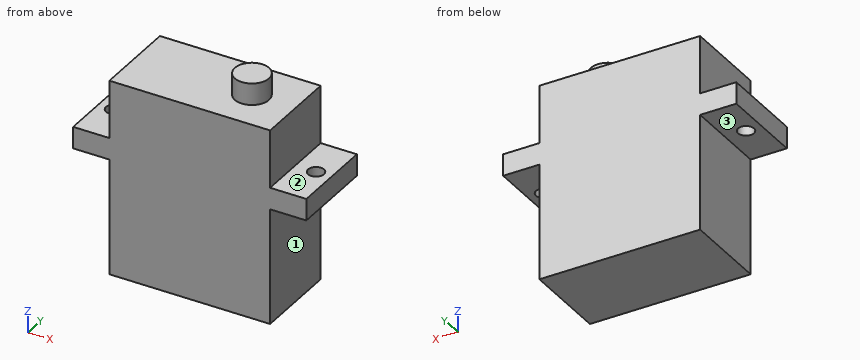
from build123d import *

# Parameters (mm, degrees)
SKETCH1_W           = 32.2
SKETCH1_H           = 11.8
BOSS_EXTRUDE1_DEPTH = 27
SKETCH2_R           = 2.365
BOSS_EXTRUDE2_DEPTH = 3
SKETCH4_W           = 16
SKETCH4_H           = 11.8
CUT_EXTRUDE1_DEPTH  = 5
SKETCH5_W           = 16
SKETCH5_H           = 11.8
CUT_EXTRUDE2_DEPTH  = 5
SKETCH6_W           = 8
SKETCH6_H           = 11.8
CUT_EXTRUDE3_DEPTH  = 5
SKETCH7_W           = 8
SKETCH7_H           = 11.8
CUT_EXTRUDE4_DEPTH  = 5
CUT_EXTRUDE5_REACH  = 21
SKETCH8_R           = 1.1


with BuildPart() as part:
    # Sketch1 → Boss-Extrude1 (new body)
    with BuildSketch(Plane.XY):
        with Locations((0, 5.9)):
            Rectangle(SKETCH1_W, SKETCH1_H)
    extrude(amount=-BOSS_EXTRUDE1_DEPTH)

    # Sketch2 → Boss-Extrude2 (add)
    with BuildSketch(Plane.XY):
        with Locations((5.1, 5.9)):
            Circle(SKETCH2_R)
    extrude(amount=BOSS_EXTRUDE2_DEPTH)

    # Sketch4 → Cut-Extrude1 (cut)
    with BuildSketch(Plane(origin=(16.1, 0, 0), x_dir=(0, 0, -1), z_dir=(1, 0, 0))):
        with Locations((19, 5.9)):
            Rectangle(SKETCH4_W, SKETCH4_H)
    extrude(amount=-CUT_EXTRUDE1_DEPTH, mode=Mode.SUBTRACT)

    # Sketch5 → Cut-Extrude2 (cut)
    with BuildSketch(Plane.ZY.offset(16.1)):
        with Locations((-19, 5.9)):
            Rectangle(SKETCH5_W, SKETCH5_H)
    extrude(amount=-CUT_EXTRUDE2_DEPTH, mode=Mode.SUBTRACT)

    # Sketch6 → Cut-Extrude3 (cut)
    with BuildSketch(Plane.ZY.offset(16.1)):
        with Locations((-4, 5.9)):
            Rectangle(SKETCH6_W, SKETCH6_H)
    extrude(amount=-CUT_EXTRUDE3_DEPTH, mode=Mode.SUBTRACT)

    # Sketch7 → Cut-Extrude4 (cut)
    with BuildSketch(Plane(origin=(16.1, 0, 0), x_dir=(0, 0, -1), z_dir=(1, 0, 0))):
        with Locations((4, 5.9)):
            Rectangle(SKETCH7_W, SKETCH7_H)
    extrude(amount=-CUT_EXTRUDE4_DEPTH, mode=Mode.SUBTRACT)

    # Sketch8 → Cut-Extrude5 (cut, up to next)
    with BuildSketch(Plane.XY.offset(-8), mode=Mode.PRIVATE) as cut_extrude5_sk1:
        with Locations((13.95, 5.9)):
            Circle(SKETCH8_R)
    cut_extrude5_tool1 = extrude(cut_extrude5_sk1.sketch, amount=-CUT_EXTRUDE5_REACH, mode=Mode.PRIVATE) & part.part
    add(cut_extrude5_tool1.solids().sort_by_distance((13.95, 5.9, -8))[0], mode=Mode.SUBTRACT)
    # Sketch8 → Cut-Extrude5 (cut, up to next)
    with BuildSketch(Plane.XY.offset(-8), mode=Mode.PRIVATE) as cut_extrude5_sk2:
        with Locations((-13.95, 5.9)):
            Circle(SKETCH8_R)
    cut_extrude5_tool2 = extrude(cut_extrude5_sk2.sketch, amount=-CUT_EXTRUDE5_REACH, mode=Mode.PRIVATE) & part.part
    add(cut_extrude5_tool2.solids().sort_by_distance((-13.95, 5.9, -8))[0], mode=Mode.SUBTRACT)


solid = part.part
Model file for the job. Use its own axes, mm. Face numbers are marked on the shaded views. A direction names the side the tool comes from. Coordinates: 2 decimals unless noted, no trailing zeros. Loops run counter-clockwise (first coordinate to the right, second up) from the corner with the lowest first, then second, coordinate; pieces in that order, holes last. Notation, with made-up numbers: (-20, 72) -> (-12, 72) arc R23 cw to (-12, 101) -> close; hole circle Ø10 at (-15, 74.25). An arc over 180 degrees is marked (long way). Use one line per item in the form item = value. Start each with the question number.
(1) Flat gauge pins, fed straight in: pin 1 (2.5 mm diameter, centred on y = 4, z = -4.5, fed in from -X); pin 2 (5.5 mm diameter, centred on x = 14.5, y = 6, fed in from +Z); pin 3 (5.5 mm diameter, centred on x = -13.5, y = 5, fed in from +Z); pin 4 (1.3 mm diameter, centred on x = -13.95, y = 5.9, fed in from -Z). Where does each tip first touch, or does it go through?
(2) Cut at C-C on x = 5.1. Give the cut face in (y, z) (3 decimals).
(3) Cut at B-B on y = 5.9. Give the cut face in (x, z) (3 decimals), and give its area (3 significant figures).
(4) Cut at A-A on x = -13.95. Give the cut face in (y, z).
(5) Tool access for the marked faces 1, 2 and 3: list every direction of +Z, -Z, +X, -X, +Y, -Y with a clear straight run to the whole face (end or side of a thin tool).
(6) Probe probe 1 along Y at (x, z) = (13.95, -9.2); probe 2 along X at (y, z) = (6.25, -10.75); probe 3 along X at (y, z) = (7.25, -14.75). List the from-to ranges inside material, lowest first. Write a range as from..to.
(7) Cut at D-D on y = 3. Give the cut face in (x, z), and give its area (3 significant figures).
Values:
q1.pin_1 = -11.1
q1.pin_2 = -8
q1.pin_3 = 0
q1.pin_4 = through
q2.outline = (0, -27) -> (11.8, -27) -> (11.8, 0) -> (8.265, 0) -> (8.265, 3) -> (3.535, 3) -> (3.535, 0) -> (0, 0) -> close
q3.outline = (-16.1, -11) -> (-15.05, -11) -> (-15.05, -8) -> (-16.1, -8) -> close; (-12.85, -11) -> (-11.1, -11) -> (-11.1, -27) -> (11.1, -27) -> (11.1, -11) -> (12.85, -11) -> (12.85, -8) -> (11.1, -8) -> (11.1, 0) -> (7.465, 0) -> (7.465, 3) -> (2.735, 3) -> (2.735, 0) -> (-11.1, 0) -> (-11.1, -8) -> (-12.85, -8) -> close; (15.05, -11) -> (16.1, -11) -> (16.1, -8) -> (15.05, -8) -> close
q3.area = 630 mm2
q4.outline = (0, -11) -> (4.8, -11) -> (4.8, -8) -> (0, -8) -> close; (7, -11) -> (11.8, -11) -> (11.8, -8) -> (7, -8) -> close
q5.face_1 = -Z, +X, +Y, -Y
q5.face_2 = +Z, +X, +Y, -Y
q5.face_3 = -Z, -X, +Y, -Y
q6.probe_1 = 0..4.8, 7..11.8
q6.probe_2 = -16.1..-14.99, -12.91..12.91, 14.99..16.1
q6.probe_3 = -11.1..11.1
q7.outline = (-16.1, -11) -> (-11.1, -11) -> (-11.1, -27) -> (11.1, -27) -> (11.1, -11) -> (16.1, -11) -> (16.1, -8) -> (11.1, -8) -> (11.1, 0) -> (-11.1, 0) -> (-11.1, -8) -> (-16.1, -8) -> close
q7.area = 629 mm2
